```python
from build123d import *

# Parameters (mm, degrees)
F0_R     = 14.345
F1_DEPTH = 53
F2_R     = 6.4
F3_DEPTH = 3
F4_R     = 1.565
F5_DEPTH = 15.35
F6_R     = 3.84
F6_R_2   = 1.565
F7_DEPTH = 10.48


with BuildPart() as f1:
    # F0 (on Front) → F1 (new body)
    with BuildSketch(Plane.XZ):
        Circle(F0_R)
    extrude(amount=F1_DEPTH)

    # F2 (on face) → F3 (join)
    with BuildSketch(Plane.XZ.offset(53)):
        Circle(F2_R)
    extrude(amount=F3_DEPTH)

    # F4 (on face) → F5 (join)
    with BuildSketch(Plane.XZ.offset(56)):
        Circle(F4_R)
    extrude(amount=F5_DEPTH)

    # F6 (on face) → F7 (join)
    with BuildSketch(Plane.XZ.offset(71.35)):
        Circle(F6_R)
        Circle(F6_R_2, mode=Mode.SUBTRACT)
    extrude(amount=-F7_DEPTH)


solid = f1.part
```
The model under review builds one solid part; all positions refer to its coordinate system, in mm. A direction names the side the tool comes from. Give positions to 0.01 mm unless a question says otherwise; leave off trailing zeros. Write each loop counter-clockwise with the first axis right and the second up, starting at its lowest first coordinate (ties: lowest second). Pieces come first, ordered by that corner, then holes.
(1) Tool access review of faces 4 (the cylindrical face through (-5.08, -54.48, -3.89)), 5 (the flat face through (1.3, -56, -1.3)), 6 (the flat face through (0, -71.35, 0)): name each direction out of +Z, -Z, +X, -X, +Y, -Y from which nothing blocks a thin tool from reaching the whole face with its end or side.
(2) Consider section D-D, the plane x = -10.5. Give the boundary of the cut face in (y, z).
(3) For P1, Ø4, axis at y = -15.5, z = -9.5, coming from the +X side; P2, Ø4, axis at y = -21, z = -8, coming from the -X side; P3, Ø12, axis at x = -10.5, y = -21.5, coming from the +Z side, all flat-tipped, find the tip position at first contact; note any pin that passes through.
(4) Consider section A-A, the plane x = 0. Give the boundary of the cut face in (y, z) (3 decimals).
(5) The part is to be moulded in two halves that separate along Y. For faces 1 (the flat face through (0, 0, 0)), 2 (the flat face through (2, -60.87, 0)), 3 (the flat face through (6, -53, -3)), say which applies: released by +Y, released by -Y, zero draft, split by the parting line, or undercut.
(6) Consider section C-C, the plane y = -49.5. Give the boundary of the cut face in (x, z) (3 decimals), and give its area (3 significant figures).
(7) To check wall thickness, follow L1, parallel to Y at x = 0, z = -7.5; L2, parallel to Z at x = 0.5, y = -9.5; L3, parallel to Z at x = 3.25, y = -31.5. State the ranges of each line that lie inside material, in increasing order.
(8) Consider section B-B, the plane z = -2.75. Give the boundary of the cut face in (x, y).
Returned:
1. face 4: -Y
1. face 5: none
1. face 6: +Z, -Z, +X, -X, -Y
2. outline: (-53, -9.77) - (0, -9.77) - (0, 9.77) - (-53, 9.77) - close
3. P1: stops at x = 12.23
3. P2: stops at x = -13.03
3. P3: stops at z = 13.62
4. outline: (-71.35, -3.84) - (-60.87, -3.84) - (-60.87, -1.565) - (-56, -1.565) - (-56, -6.4) - (-53, -6.4) - (-53, -14.345) - (0, -14.345) - (0, 14.345) - (-53, 14.345) - (-53, 6.4) - (-56, 6.4) - (-56, 1.565) - (-60.87, 1.565) - (-60.87, 3.84) - (-71.35, 3.84) - close
5. face 1: released by +Y
5. face 2: undercut
5. face 3: released by -Y
6. outline: circle Ø28.69 at (0, 0)
6. area: 646 mm2
7. L1: y = -53 to 0
7. L2: z = -14.34 to 14.34
7. L3: z = -13.97 to 13.97
8. outline: (-14.08, -53) - (-5.78, -53) - (-5.78, -56) - (5.78, -56) - (5.78, -53) - (14.08, -53) - (14.08, 0) - (-14.08, 0) - close; (-2.68, -71.35) - (2.68, -71.35) - (2.68, -60.87) - (-2.68, -60.87) - close
